The drawing under review shows one solid part. Ordinate dimensions are in mm from its lowest x, y, z. Give positions to 0.01 mm unless a question says otherwise; leave off trailing zeros. Write each loop counter-clockwise with the first axis right and the second up, starting at its lowest first coordinate (ties: lowest second). Pieces come first, ordered by that corner, then holes. Notation, with made-up numbers: M 20,65 L 78,65 A26 cw 78,88 Z; hole C -4,54.25 d4. An arc over 180 degrees is marked long. Use one line per item in the form item = value. Start each with the question number.
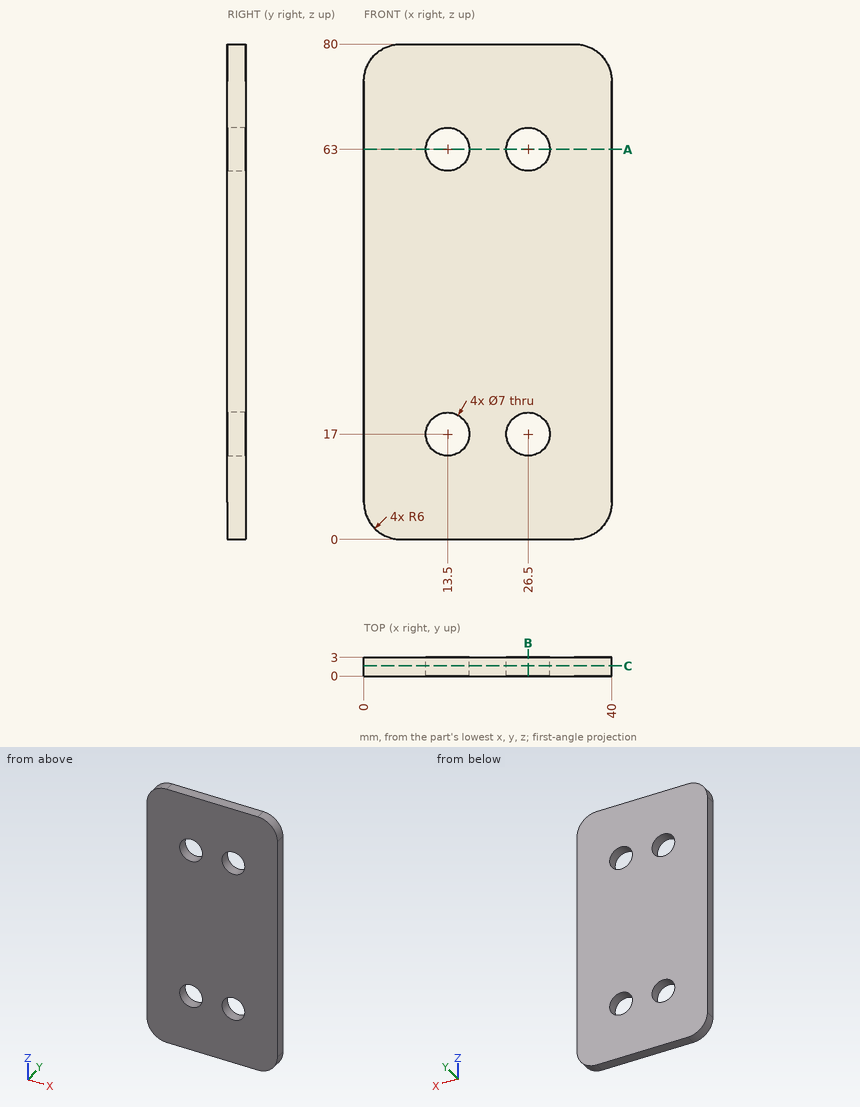
1. To check wall thickness, follow L1, parallel to X at y = 2.3, z = 63; L2, parallel to X at y = 1.6, z = 14; L3, parallel to Z at x = 38.5, y = 1.5. State the ranges of each line that lie inside material, in increasing order.
2. Clearance check with a flat-ended pin moving along its axis: pin 1 Ø6.5 at (x, z) = (13.5, 17) entering from -Y. State where the tip first meets the part, or that it passes through.
3. We need section B-B (x = 26.5). State the section outline as (y, z) points.
4. We need section A-A (z = 63). State the section outline as (x, y) points.
5. We need section C-C (y = 1.65). State the section outline as (x, z) points, and give its area (3 significant figures).
Answer block:
q1.L1 = 0 to 10, 17 to 23, 30 to 40
q1.L2 = 0 to 11.7, 15.3 to 24.7, 28.3 to 40
q1.L3 = 2.03 to 77.97
q2.pin_1 = through
q3.outline = M 0,0 L 3,0 L 3,13.5 L 0,13.5 Z; M 0,20.5 L 3,20.5 L 3,59.5 L 0,59.5 Z; M 0,66.5 L 3,66.5 L 3,80 L 0,80 Z
q4.outline = M 0,0 L 10,0 L 10,3 L 0,3 Z; M 17,0 L 23,0 L 23,3 L 17,3 Z; M 30,0 L 40,0 L 40,3 L 30,3 Z
q5.outline = M 0,6 A6 ccw 6,0 L 34,0 A6 ccw 40,6 L 40,74 A6 ccw 34,80 L 6,80 A6 ccw 0,74 Z; hole C 13.5,17 d7; hole C 13.5,63 d7; hole C 26.5,17 d7; hole C 26.5,63 d7
q5.area = 3,020 mm^2
